Work out the finished part from the listing and answer in its coordinate system (mm). A direction names the side the tool comes from. Coordinates: 2 decimals unless noted, no trailing zeros. Order: outer loops, then holes, each group sorted by start corner. A loop starts at its lowest first (then second) coordinate and runs counter-clockwise, first axis right, second up. Notation, with made-up numbers: M 81,-10 L 101,-10 A19 ccw 101,22 Z; hole C 25,-38 d2. An arc over 180 degrees is marked long. Use a Markdown table: item, result.
from build123d import *

# Parameters (mm, degrees)
F0_W     = 25.4
F0_H     = 15.875
F1_DEPTH = 22.225
F2_T     = -1.5875
F3_W     = 23.8125
F3_H     = 14.2875
F4_DEPTH = 19.5326
F5_R     = 1.5875
F6_R     = 1.5875


with BuildPart() as f1:
    # F0 (on Front) → F1 (new body, symmetric)
    with BuildSketch(Plane.XZ):
        Rectangle(F0_W, F0_H)
    extrude(amount=F1_DEPTH, both=True)

    # F2
    f2_openings = [f1.faces().sort_by_distance(p)[0] for p in [
        (0, -22.225, 0),
        (0, 22.225, 0),
    ]]
    offset(amount=F2_T, openings=f2_openings)

    # F3 (on Front) → F4 (join, symmetric)
    with BuildSketch(Plane.XZ):
        Rectangle(F3_W, F3_H)
    extrude(amount=F4_DEPTH, both=True)

    # F5
    f5_edges = [f1.edges().sort_by_distance(p)[0] for p in [
        (-11.1125, -20.8788, 6.35),
        (11.1125, -20.8788, 6.35),
        (11.1125, -20.8788, -6.35),
        (-11.1125, -20.8788, -6.35),
        (-11.1125, 20.8788, -6.35),
        (11.1125, 20.8788, -6.35),
        (-11.1125, 20.8788, 6.35),
        (11.1125, 20.8788, 6.35),
    ]]
    fillet(f5_edges, radius=F5_R)

    # F6
    f6_edges = [f1.edges().sort_by_distance(p)[0] for p in [
        (-12.7, 0, -7.9375),
        (-12.7, 0, 7.9375),
        (12.7, 0, 7.9375),
        (12.7, 0, -7.9375),
    ]]
    fillet(f6_edges, radius=F6_R)


solid = f1.part
(1) Given P1, Ø6, axis at x = 6, z = 1.5, coming from the +Y side; P2, Ø3, axis at x = 6.5, z = 3, coming from the -Y side; P3, Ø6, axis at x = 0, z = -5, coming from the +Y side (3 decimals), each flat-ended and moving along its own axis, determine where each tip first touches the part or whether it passes through.
Conclusion:
| item | result |
|---|---|
| P1 | y = 19.53 |
| P2 | y = -19.53 |
| P3 | y = 22.225 |
(2) Determine the mould class of faces 1 (the cylindrical face through (-12.25, -0.31, -7.46)), 2 (the cylindrical face through (-10.635, -20.86, -5.897)), 3 (the cylindrical face through (12.223, -0.311, -7.485)), 4 (the cylindrical face through (-10.635, 20.898, -5.897)) for opening direction X: pulls with the +X half, pulls with the -X half, needs draft (parallel to the pull), parting line crosses it, or undercut.
Conclusion:
| item | result |
|---|---|
| face 1 | pulls with the -X half |
| face 2 | undercut |
| face 3 | pulls with the +X half |
| face 4 | undercut |
(3) Straight lines are drawn through the part: L1, parallel to Y at x = 7.5, z = -6.25; L2, parallel to Z at x = -5.5, y = 20.5; L3, parallel to X at y = 19, z = -7. For each, find the intervals that lie inside material, in ascending order.
Conclusion:
| item | result |
|---|---|
| L1 | -19.53 to 19.53 |
| L2 | -7.94 to -6.35, 6.35 to 7.94 |
| L3 | -12.56 to 12.56 |
(4) A cutting plane is placed at B-B (z = -1). Determine the outline of the cut face in (x, y) (1 decimal), then the cut area to 3 significant figures.
Conclusion:
| item | result |
|---|---|
| outline | M -12.7,-22.2 L -11.1,-22.2 L -11.1,-19.5 L 11.1,-19.5 L 11.1,-22.2 L 12.7,-22.2 L 12.7,22.2 L 11.1,22.2 L 11.1,19.5 L -11.1,19.5 L -11.1,22.2 L -12.7,22.2 Z |
| area | 1,010 mm2 |
(5) Which of the six approach directions +Z, -Z, +X, -X, +Y, -Y give full straight-line access (tool end or side, diameter ignored) to faces 5 (the cylindrical face through (10.635, 20.898, 5.897)), 6 (the flat face through (12.7, 0, 0)), 7 (the flat face through (11.112, -21, 0))?
Conclusion:
| item | result |
|---|---|
| face 5 | +Y |
| face 6 | +Z, -Z, +X, +Y, -Y |
| face 7 | -Y |
